from build123d import *

# Parameters (mm, degrees)
SKETCH_1_R      = 1.5
SKETCH_1_R_2    = 2.5
SKETCH_1_R_3    = 1.55
SKETCH_1_R_4    = 1.25
SKETCH_1_R_5    = 1
EXTRUDE_1_DEPTH = 1.5


with BuildPart() as part:
    # 草图1 → 凸台-拉伸1 (new, symmetric)
    with BuildSketch(Plane(origin=(0, 0, 0), x_dir=(1, 0, 0), z_dir=(0, 1, 0))):
        with BuildLine():
            Line((132, -5), (132, -25))
            ThreePointArc((132, -25), (130.535533906, -28.535533906), (127, -30))
            Line((127, -30), (75, -30))
            ThreePointArc((75, -30), (71.464466094, -28.535533906), (70, -25))
            Line((70, -25), (70, -5))
            ThreePointArc((70, -5), (68.535533906, -1.464466094), (65, 0))
            Line((65, 0), (7.5, 0))
            ThreePointArc((7.5, 0), (2.196699141, 2.196699141), (0, 7.5))
            Line((0, 7.5), (0, 95))
            ThreePointArc((0, 95), (2.196699141, 100.303300859), (7.5, 102.5))
            Line((7.5, 102.5), (65, 102.5))
            ThreePointArc((65, 102.5), (68.535533906, 103.964466094), (70, 107.5))
            Line((70, 107.5), (70, 127.5))
            ThreePointArc((70, 127.5), (71.464466094, 131.035533906), (75, 132.5))
            Line((75, 132.5), (127, 132.5))
            ThreePointArc((127, 132.5), (130.535533906, 131.035533906), (132, 127.5))
            Line((132, 127.5), (132, 107.5))
            ThreePointArc((132, 107.5), (133.464466094, 103.964466094), (137, 102.5))
            Line((137, 102.5), (178.395701384, 102.5))
            ThreePointArc((178.395701384, 102.5), (192.537837007, 96.642135624), (198.395701384, 82.5))
            Line((198.395701384, 82.5), (198.395701384, 20))
            ThreePointArc((198.395701384, 20), (192.537837007, 5.857864376), (178.395701384, 0))
            Line((178.395701384, 0), (137, 0))
            ThreePointArc((137, 0), (133.464466094, -1.464466094), (132, -5))
        make_face()
        with Locations(Location((96.855482095, 24.5, 0), (0, 0, 270))):
            Circle(SKETCH_1_R, mode=Mode.SUBTRACT)
        with Locations(Location((135.355482095, 24.5, 0), (0, 0, 270))):
            Circle(SKETCH_1_R, mode=Mode.SUBTRACT)
        with Locations(Location((65.477875917, 19.059382071, 0), (0, 0, 270))):
            Circle(SKETCH_1_R_2, mode=Mode.SUBTRACT)
        with Locations(Location((30, 41.5, 0), (0, 0, 270))):
            Circle(SKETCH_1_R_3, mode=Mode.SUBTRACT)
        with Locations(Location((140.705086193, 36.25, 0), (0, 0, 270))):
            Circle(SKETCH_1_R_4, mode=Mode.SUBTRACT)
        with Locations(Location((164.705086193, 36.25, 0), (0, 0, 270))):
            Circle(SKETCH_1_R_4, mode=Mode.SUBTRACT)
        with Locations(Location((79.074216313, -16.098364995, 0), (0, 0, 270))):
            Circle(SKETCH_1_R_3, mode=Mode.SUBTRACT)
        with Locations(Location((121.803446989, -16.098364995, 0), (0, 0, 270))):
            Circle(SKETCH_1_R_3, mode=Mode.SUBTRACT)
        with Locations(Location((50, 10, 0), (0, 0, 270))):
            Circle(SKETCH_1_R_5, mode=Mode.SUBTRACT)
        with Locations(Location((164.705086193, 66.25, 0), (0, 0, 90))):
            Circle(SKETCH_1_R_4, mode=Mode.SUBTRACT)
        with Locations(Location((140.705086193, 66.25, 0), (0, 0, 90))):
            Circle(SKETCH_1_R_4, mode=Mode.SUBTRACT)
        with Locations(Location((135.355482095, 78, 0), (0, 0, 90))):
            Circle(SKETCH_1_R, mode=Mode.SUBTRACT)
        with Locations(Location((96.855482095, 78, 0), (0, 0, 90))):
            Circle(SKETCH_1_R, mode=Mode.SUBTRACT)
        with Locations(Location((65.477875917, 83.440617929, 0), (0, 0, 90))):
            Circle(SKETCH_1_R_2, mode=Mode.SUBTRACT)
        with Locations(Location((50, 92.5, 0), (0, 0, 90))):
            Circle(SKETCH_1_R_5, mode=Mode.SUBTRACT)
        with Locations(Location((30, 61, 0), (0, 0, 90))):
            Circle(SKETCH_1_R_3, mode=Mode.SUBTRACT)
        with Locations(Location((55, 10, 0), (0, 0, 270))):
            Circle(SKETCH_1_R_5, mode=Mode.SUBTRACT)
        with Locations(Location((55, 92.5, 0), (0, 0, 90))):
            Circle(SKETCH_1_R_5, mode=Mode.SUBTRACT)
        with Locations(Location((121.803446989, 118.598364995, 0), (0, 0, 90))):
            Circle(SKETCH_1_R_3, mode=Mode.SUBTRACT)
        with Locations(Location((79.074216313, 118.598364995, 0), (0, 0, 90))):
            Circle(SKETCH_1_R_3, mode=Mode.SUBTRACT)
        with Locations(Location((191.545701384, 36.25, 0), (0, 0, 270))):
            Circle(SKETCH_1_R_3, mode=Mode.SUBTRACT)
        with Locations(Location((191.545701384, 66.25, 0), (0, 0, 90))):
            Circle(SKETCH_1_R_3, mode=Mode.SUBTRACT)
    extrude(amount=EXTRUDE_1_DEPTH, both=True)


solid = part.part
Read the model definition and answer for the solid it produces. Units are mm, in the model's axes. Coordinates: 2 decimals unless noted, no trailing zeros. Loops run counter-clockwise (first coordinate to the right, second up) from the corner with the lowest first, then second, coordinate; pieces in that order, holes last. Notation, with made-up numbers: (37, 89.25) -> (46, 89.25) arc R26 cw to (46, 128.25) -> close; hole circle Ø2 at (8.5, -13.75). An arc over 180 degrees is marked (long way). Write item = value, one per line. Start each with the question number.
1) Find the intervals of material crossed by L1, parallel to X at y = -0.75, z = -66.25; L2, parallel to X at y = 0.3, z = -78; L3, parallel to X at y = -0.55, z = -61, in increasing order. Write a range as from..to.
2) The mould has two halves that part along X. Classify faces 1 (the face through (131, 0, 28)), 2 (the face through (101, -1.5, -52)), 3 (the face through (66.999, -0.021, -81.457)): pulls with the +X half, pulls with the -X half, needs draft (parallel to the pull), parting line crosses it, or undercut.
3) The part is cut by section B-B, the plane y = 0.15. State how many separate pieces and enclosed holes the cut face has, plus the area to 3 significant figures.
4) The part is cut by section A-A, the plane x = 147. Determine the outline of the cut face in (y, z).
5) Given P1, Ø1.5, axis at y = 0.5, z = 16.5, coming from the -X side; P2, Ø1.5, axis at x = 156.5, y = -0.5, coming from the -Z side, each flat-ended and moving along its own axis, determine where each tip first touches the part or whether it passes through.
Result:
q1.L1 = 0..139.46, 141.96..163.46, 165.96..190, 193.1..198.4
q1.L2 = 0..95.36, 98.36..133.86, 136.86..198.4
q1.L3 = 0..28.45, 31.55..198.4
q2.face_1 = pulls with the +X half
q2.face_2 = needs draft
q2.face_3 = undercut
q3.separate_pieces = 1
q3.enclosed_holes = 22
q3.area = 23,700 mm²
q4.outline = (-1.5, -102.5) -> (1.5, -102.5) -> (1.5, 0) -> (-1.5, 0) -> close
q5.P1 = 70
q5.P2 = -102.5
